Here's how the part is built. I have some questions about the finished solid (model axes, mm). A direction names the side the tool comes from. Coordinates: 2 decimals unless noted, no trailing zeros. Write each loop counter-clockwise with the first axis right and the second up, starting at its lowest first coordinate (ties: lowest second). Pieces come first, ordered by that corner, then holes. Notation, with made-up numbers: M -25.75,65.25 L 26.25,65.25 A17 cw 26.25,93.25 Z; hole C -22.5,16.25 d1. An arc over 180 degrees is marked long. Use a Markdown table: item, result.
```python
from build123d import *

# Parameters (mm, degrees)
SKETCH1_W            = 72.7
SKETCH1_H            = 61
BOSS_EXTRUDE1_DEPTH  = 1.5
SKETCH3_W            = 76.7
SKETCH3_H            = 65
BOSS_EXTRUDE5_DEPTH  = 1.5
SKETCH2_W            = 76.7
SKETCH2_H            = 65
BOSS_EXTRUDE6_DEPTH  = 4.2
SKETCH4_W            = 76.7
SKETCH4_H            = 65
BOSS_EXTRUDE7_DEPTH  = 3.8
SKETCH5_W            = 76.7
SKETCH5_H            = 65
BOSS_EXTRUDE8_DEPTH  = 8.5
SKETCH7_R            = 1.1
CUT_EXTRUDE1_DEPTH   = 20.8
FILLET3_R            = 8
SKETCH9_W            = 1.2
SKETCH9_H            = 4
CUT_EXTRUDE2_DEPTH   = 8
BOSS_EXTRUDE11_DEPTH = 4.2
FILLET4_R            = 6
FILLET2_R            = 8
BOSS_EXTRUDE12_DEPTH = 18
BOSS_EXTRUDE13_DEPTH = 0.3
SKETCH14_R           = 1.1
CUT_EXTRUDE3_DEPTH   = 14


with BuildPart() as part:
    # Sketch1 → Boss-Extrude1 (new body)
    with BuildSketch(Plane(origin=(0, 0, 0), x_dir=(1, 0, 0), z_dir=(0, 1, 0))):
        Rectangle(SKETCH1_W, SKETCH1_H)
    extrude(amount=BOSS_EXTRUDE1_DEPTH)

    # Sketch3 → Boss-Extrude5 (add)
    with BuildSketch(Plane.XZ):
        Rectangle(SKETCH3_W, SKETCH3_H)
    extrude(amount=-BOSS_EXTRUDE5_DEPTH)

    # Sketch2 → Boss-Extrude6 (add)
    with BuildSketch(Plane(origin=(0, 1.5, 0), x_dir=(1, 0, 0), z_dir=(0, 1, 0))):
        Rectangle(SKETCH2_W, SKETCH2_H)
        Polygon((-2.65, 30.5), (-2.65, 26.1), (-2.65, 22.1), (-3.85, 22.1), (-3.85, 26.1), (-17.95, 26.1), (-17.95, 22.1), (-36.35, 22.1), (-36.35, -22.1), (-17.95, -22.1), (-17.95, -26.1), (-3.85, -26.1), (-3.85, -22.1), (-2.65, -22.1), (-2.65, -26.1), (-2.65, -30.5), (36.35, -30.5), (36.35, 30.5), align=None, mode=Mode.SUBTRACT)
    extrude(amount=BOSS_EXTRUDE6_DEPTH)

    # Sketch4 → Boss-Extrude7 (add)
    with BuildSketch(Plane(origin=(0, 5.7, 0), x_dir=(1, 0, 0), z_dir=(0, 1, 0))):
        Rectangle(SKETCH4_W, SKETCH4_H)
        Polygon((-36.35, -22.1), (-36.35, -23.2), (-17.95, -23.2), (-17.95, -26.1), (-3.85, -26.1), (-3.85, -22.1), (-2.65, -22.1), (-2.65, -30.5), (36.35, -30.5), (36.35, 30.5), (-2.65, 30.5), (-2.65, 22.1), (-3.85, 22.1), (-3.85, 26.1), (-17.95, 26.1), (-17.95, 23.2), (-36.35, 23.2), (-36.35, 22.1), align=None, mode=Mode.SUBTRACT)
    extrude(amount=BOSS_EXTRUDE7_DEPTH)

    # Sketch5 → Boss-Extrude8 (add)
    with BuildSketch(Plane(origin=(0, 9.5, 0), x_dir=(1, 0, 0), z_dir=(0, 1, 0))):
        Rectangle(SKETCH5_W, SKETCH5_H)
        Polygon((-2.65, -27.8), (-3.85, -27.8), (-7.15, -27.8), (-7.15, -26.1), (-17.95, -26.1), (-17.95, -23.2), (-36.35, -23.2), (-36.35, 23.2), (-17.95, 23.2), (-17.95, 26.1), (-7.15, 26.1), (-7.15, 27.8), (-3.85, 27.8), (-2.65, 27.8), (-2.65, 30.5), (36.35, 30.5), (36.35, -30.5), (-2.65, -30.5), align=None, mode=Mode.SUBTRACT)
    extrude(amount=BOSS_EXTRUDE8_DEPTH)

    # Sketch7 → Cut-Extrude1 (cut)
    with BuildSketch(Plane(origin=(0, 0, 23.2), x_dir=(-1, 0, 0), z_dir=(0, 0, -1))):
        with Locations((27.35, 10.5)):
            Circle(SKETCH7_R)
    extrude(amount=-CUT_EXTRUDE1_DEPTH, mode=Mode.SUBTRACT)

    # Fillet3
    fillet3_edges = [part.edges().sort_by_distance(p)[0] for p in [
        (-38.35, 9, -32.5),
        (-38.35, 9, 32.5),
    ]]
    fillet(fillet3_edges, radius=FILLET3_R)

    # Sketch9 → Cut-Extrude2 (cut)
    with BuildSketch(Plane(origin=(0, 9.5, 0), x_dir=(1, 0, 0), z_dir=(0, 1, 0))):
        with Locations((-3.25, 24.1)):
            Rectangle(SKETCH9_W, SKETCH9_H)
        with Locations((-3.25, -24.1)):
            Rectangle(SKETCH9_W, SKETCH9_H)
    extrude(amount=-CUT_EXTRUDE2_DEPTH, mode=Mode.SUBTRACT)

    # Sketch11 → Boss-Extrude11 (add)
    with BuildSketch(Plane(origin=(0, 1.5, 0), x_dir=(1, 0, 0), z_dir=(0, 1, 0))):
        Polygon((-16.85, -22.1), (-17.95, -22.1), (-17.95, -26.1), (-2.65, -26.1), (-2.65, -25), (-16.85, -25), align=None)
        Polygon((-17.95, 26.1), (-17.95, 22.1), (-16.85, 22.1), (-16.85, 25), (-2.65, 25), (-2.65, 26.1), align=None)
    extrude(amount=BOSS_EXTRUDE11_DEPTH)

    # Fillet4
    fillet4_edges = [part.edges().sort_by_distance(p)[0] for p in [
        (36.35, 9.75, -30.5),
        (36.35, 9.75, 30.5),
    ]]
    fillet(fillet4_edges, radius=FILLET4_R)

    # Fillet2
    fillet2_edges = [part.edges().sort_by_distance(p)[0] for p in [
        (38.35, 9, -32.5),
        (38.35, 9, 32.5),
    ]]
    fillet(fillet2_edges, radius=FILLET2_R)

    # Sketch12 → Boss-Extrude12 (add)
    with BuildSketch(Plane(origin=(0, 18, 0), x_dir=(1, 0, 0), z_dir=(0, 1, 0))):
        with BuildLine():
            Line((-30.35, -33), (30.35, -33))
            ThreePointArc((30.35, -33), (36.36040764, -30.51040764), (38.85, -24.5))
            Line((38.85, -24.5), (38.85, 24.5))
            ThreePointArc((38.85, 24.5), (36.36040764, 30.51040764), (30.35, 33))
            Line((30.35, 33), (-30.35, 33))
            ThreePointArc((-30.35, 33), (-36.36040764, 30.51040764), (-38.85, 24.5))
            Line((-38.85, 24.5), (-38.85, -24.5))
            ThreePointArc((-38.85, -24.5), (-36.36040764, -30.51040764), (-30.35, -33))
        make_face()
        with BuildLine():
            Line((38.35, -24.5), (38.35, 24.5))
            ThreePointArc((38.35, 24.5), (36.006854249, 30.156854249), (30.35, 32.5))
            Line((30.35, 32.5), (-30.35, 32.5))
            ThreePointArc((-30.35, 32.5), (-36.006854249, 30.156854249), (-38.35, 24.5))
            Line((-38.35, 24.5), (-38.35, -24.5))
            ThreePointArc((-38.35, -24.5), (-36.006854249, -30.156854249), (-30.35, -32.5))
            Line((-30.35, -32.5), (30.35, -32.5))
            ThreePointArc((30.35, -32.5), (36.006854249, -30.156854249), (38.35, -24.5))
        make_face(mode=Mode.SUBTRACT)
    extrude(amount=-BOSS_EXTRUDE12_DEPTH)

    # Sketch13 → Boss-Extrude13 (add)
    with BuildSketch(Plane(origin=(0, 18, 0), x_dir=(1, 0, 0), z_dir=(0, 1, 0))):
        with BuildLine():
            Line((-30.35, -31.5), (30.35, -31.5))
            ThreePointArc((30.35, -31.5), (35.299747468, -29.449747468), (37.35, -24.5))
            Line((37.35, -24.5), (37.35, 24.5))
            ThreePointArc((37.35, 24.5), (35.299747468, 29.449747468), (30.35, 31.5))
            Line((30.35, 31.5), (-30.35, 31.5))
            ThreePointArc((-30.35, 31.5), (-35.299747468, 29.449747468), (-37.35, 24.5))
            Line((-37.35, 24.5), (-37.35, -24.5))
            ThreePointArc((-37.35, -24.5), (-35.299747468, -29.449747468), (-30.35, -31.5))
        make_face()
        with BuildLine():
            Line((-36.95, 24.5), (-36.95, -24.5))
            ThreePointArc((-36.95, -24.5), (-35.016904756, -29.166904756), (-30.35, -31.1))
            Line((-30.35, -31.1), (30.35, -31.1))
            ThreePointArc((30.35, -31.1), (35.016904756, -29.166904756), (36.95, -24.5))
            Line((36.95, -24.5), (36.95, 24.5))
            ThreePointArc((36.95, 24.5), (35.016904756, 29.166904756), (30.35, 31.1))
            Line((30.35, 31.1), (-30.35, 31.1))
            ThreePointArc((-30.35, 31.1), (-35.016904756, 29.166904756), (-36.95, 24.5))
        make_face(mode=Mode.SUBTRACT)
    extrude(amount=BOSS_EXTRUDE13_DEPTH)

    # Sketch14 → Cut-Extrude3 (cut)
    with BuildSketch(Plane(origin=(0, 0, 23.2), x_dir=(-1, 0, 0), z_dir=(0, 0, -1))):
        with Locations((27.35, 10.5)):
            Circle(SKETCH14_R)
    extrude(amount=-CUT_EXTRUDE3_DEPTH, mode=Mode.SUBTRACT)


solid = part.part
```
1. Suppose I cut it at C-C on z = -2. Write out the boundary of the cut face in (x, y), and give its area (3 significant figures).
Answers follow:
| item | result |
|---|---|
| outline | M -38.85,0 L 38.85,0 L 38.85,18 L 37.35,18 L 37.35,18.3 L 36.95,18.3 L 36.95,18 L 36.35,18 L 36.35,1.5 L -36.35,1.5 L -36.35,18 L -36.95,18 L -36.95,18.3 L -37.35,18.3 L -37.35,18 L -38.85,18 Z |
| area | 199 mm2 |
2. I need wall thicknesses on probe 1 along Z at (x, y) = (26, 14.5); probe 2 along X at (y, z) = (17, -1); probe 3 along Y at (x, z) = (-27.35, 29.75). Which ranges of each line are inside material? Lowest first, please.
Answers follow:
| item | result |
|---|---|
| probe 1 | z = -33 to -30.5, 30.5 to 33 |
| probe 2 | x = -38.85 to -36.35, 36.35 to 38.85 |
| probe 3 | y = 0 to 9.4, 11.6 to 18 |
3. Will these pins go through, and if not, where does the flat tip stop? pin 1 Ø0.5 at (x, z) = (-4, -26.5) entering from +Y; pin 2 Ø1.4 at (y, z) = (12, 27) entering from +X; pin 3 Ø4 at (x, z) = (7.5, -6.5) entering from +Y.
Answers follow:
| item | result |
|---|---|
| pin 1 | stops at y = 9.5 |
| pin 2 | stops at x = 38.66 |
| pin 3 | stops at y = 1.5 |
4. We'd pull the mould along X, two halves only. Please class faces 1 (the face through (-36.43, 9.13, 30.44)), 2 (the face through (-7.15, 14, 27)), 3 (the face through (0, 9, 33)): +X half, -X half, draft (parallel to the pull), parting line (faces both ways), or undercut.
Answers follow:
| item | result |
|---|---|
| face 1 | -X half |
| face 2 | undercut |
| face 3 | draft |
5. Suppose I cut it at A-A on x = -27.35. Write out the boundary of the cut face in (y, z).
Answers follow:
| item | result |
|---|---|
| outline | M 0,-33 L 18,-33 L 18,-31.5 L 18.3,-31.5 L 18.3,-31.1 L 18,-31.1 L 18,-23.2 L 5.7,-23.2 L 5.7,-22.1 L 1.5,-22.1 L 1.5,22.1 L 5.7,22.1 L 5.7,23.2 L 9.4,23.2 L 9.4,33 L 0,33 Z; M 11.6,23.2 L 18,23.2 L 18,31.1 L 18.3,31.1 L 18.3,31.5 L 18,31.5 L 18,33 L 11.6,33 Z |
6. Which directions (+Z, -Z, +X, -X, +Y, -Y) give clear straight access to the entire face, cutting with the end or side of a thin tool? Please do faces 4 (the face through (-28.366, 10.079, 28.031)), 5 (the face through (-38.85, 9, 0)), 6 (the face through (-5, 9.5, 27)).
Answers follow:
| item | result |
|---|---|
| face 4 | +Z |
| face 5 | +Z, -Z, -X, +Y, -Y |
| face 6 | +Y |
7. Suppose I cut it at B-B on y = 12.75. Write out the boundary of the cut face in (x, z).
Answers follow:
| item | result |
|---|---|
| outline | M -38.85,-24.5 A8.5 ccw -30.35,-33 L 30.35,-33 A8.5 ccw 38.85,-24.5 L 38.85,24.5 A8.5 ccw 30.35,33 L -30.35,33 A8.5 ccw -38.85,24.5 Z; hole M -36.35,-23.2 L -17.95,-23.2 L -17.95,-26.1 L -7.15,-26.1 L -7.15,-27.8 L -2.65,-27.8 L -2.65,-30.5 L 30.35,-30.5 A6 ccw 36.35,-24.5 L 36.35,24.5 A6 ccw 30.35,30.5 L -2.65,30.5 L -2.65,27.8 L -7.15,27.8 L -7.15,26.1 L -17.95,26.1 L -17.95,23.2 L -36.35,23.2 Z |
8. Suppose I cut it at D-D on x = 8. Write out the boundary of the cut face in (y, z).
Answers follow:
| item | result |
|---|---|
| outline | M 0,-33 L 18,-33 L 18,-31.5 L 18.3,-31.5 L 18.3,-31.1 L 18,-31.1 L 18,-30.5 L 1.5,-30.5 L 1.5,30.5 L 18,30.5 L 18,31.1 L 18.3,31.1 L 18.3,31.5 L 18,31.5 L 18,33 L 0,33 Z |
